```python
from build123d import *

# Parameters (mm, degrees)
SKETCH2_W                        = 127
SKETCH2_H                        = 50.8
BOSS_EXTRUDE1_DEPTH              = 11.43
FILLET1_R                        = 6.35
F_17_64_0_26563_DIAMETER_HOLE2_D = 6.747002
F_17_64_0_26563_DIAMETER_HOLE3_D = 6.747002
F_17_64_0_26563_DIAMETER_HOLE4_D = 6.747002
F_17_64_0_26563_DIAMETER_HOLE6_D = 6.747002


with BuildPart() as part:
    # Sketch2 → Boss-Extrude1 (new body)
    with BuildSketch(Plane.XY):
        with Locations((15.383424408, -0.971584699)):
            Rectangle(SKETCH2_W, SKETCH2_H)
    extrude(amount=BOSS_EXTRUDE1_DEPTH)

    # Fillet1
    fillet1_edges = [part.edges().sort_by_distance(p)[0] for p in [
        (-48.116575592, 24.428415301, 5.715),
        (-48.116575592, -26.371584699, 5.715),
    ]]
    fillet(fillet1_edges, radius=FILLET1_R)

    # 17/64 (0.26563) Diameter Hole2 (through all)
    with Locations(Plane(origin=(52.213424408, 15.538415301, 0), x_dir=(-1, 0, 0), z_dir=(0, 0, -1))):
        with Locations((0, 0), (33.02, 0), (33.02, -33.02), (0, -33.02)):
            Hole(F_17_64_0_26563_DIAMETER_HOLE2_D / 2)

    # 17/64 (0.26563) Diameter Hole3 (through all)
    with Locations(Plane(origin=(-16.366575592, 14.903415301, 0), x_dir=(-1, 0, 0), z_dir=(0, 0, -1))):
        with Locations((0, 0), (0, -31.75)):
            Hole(F_17_64_0_26563_DIAMETER_HOLE3_D / 2)

    # 17/64 (0.26563) Diameter Hole4 (through all)
    with Locations(Plane(origin=(72.850924408, -16.846584699, 0), x_dir=(-1, 0, 0), z_dir=(0, 0, -1))):
        with Locations((0, 0), (0, 31.75)):
            Hole(F_17_64_0_26563_DIAMETER_HOLE4_D / 2)

    # 17/64 (0.26563) Diameter Hole6 (through all)
    with Locations(Plane(origin=(-29.066575592, 18.078415301, 0), x_dir=(-1, 0, 0), z_dir=(0, 0, -1))):
        with Locations((0, 0), (12.7, 0), (12.7, -38.1), (0, -38.1)):
            Hole(F_17_64_0_26563_DIAMETER_HOLE6_D / 2)


solid = part.part
```
Verification items for the finished model (mm, model axes). Give positions to 0.01 mm unless a question says otherwise; leave off trailing zeros.
1. Thickness scan on line 1 (Y direction, x = -41.5, z = 9.75); line 2 (Y direction, x = 20, z = 7.25); line 3 (X direction, y = 12.5, z = 1.5). Record the ranges inside material, lowest first.
2. Section check A-A, the plane z = 8.5. Count the separate pieces of the cut face and the enclosed holes in it, then the cut area to 3 significant figures.
3. Mould release check, pull along Y, two halves, no side actions. Record for faces 1 (the flat face through (18, 24.428, 6)), 2 (the flat face through (78.883, -1, 6)), 3 (the cylindrical face through (18.754, 18.883, 5.795)): released by +Y, released by -Y, zero draft, split by the parting line, or undercut.
Geometry says:
1. line 1: y = -26.37 to -23.38, -16.66 to 14.72, 21.44 to 24.43
1. line 2: y = -26.37 to -20.76, -14.21 to 12.26, 18.81 to 24.43
1. line 3: x = -48.12 to -18.73, -14 to 17.73, 20.66 to 50.75, 53.68 to 70.48, 75.22 to 78.88
2. separate pieces: 1
2. enclosed holes: 12
2. area: 6,010 mm2
3. face 1: released by +Y
3. face 2: zero draft
3. face 3: undercut
